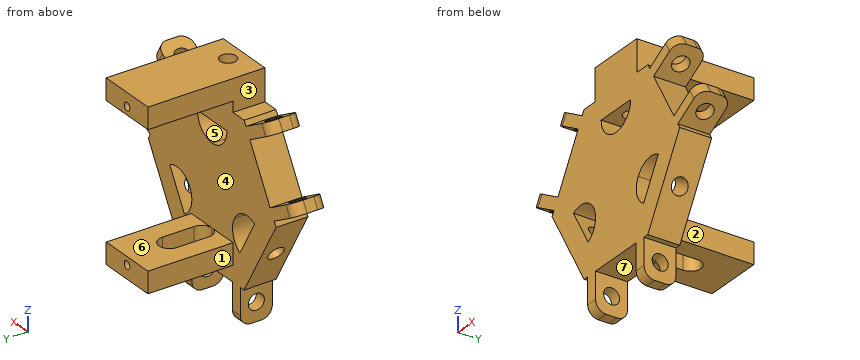
from build123d import *

# Parameters (mm, degrees)
BOSS_EXTRUDE1_DEPTH = 6
SKETCH2_W           = 2.16
SKETCH2_H           = 6
BOSS_EXTRUDE2_DEPTH = 7
SKETCH4_W           = 2.16
SKETCH4_H           = 6
BOSS_EXTRUDE3_DEPTH = 7
SKETCH5_W           = 2.16
SKETCH5_H           = 6
BOSS_EXTRUDE4_DEPTH = 7
SKETCH6_W           = 2.16
SKETCH6_H           = 6
BOSS_EXTRUDE5_DEPTH = 7
SKETCH7_W           = 2.16
SKETCH7_H           = 6
BOSS_EXTRUDE6_DEPTH = 7
SKETCH9_W           = 2.16
SKETCH9_H           = 6
BOSS_EXTRUDE7_DEPTH = 7
SKETCH11_W          = 11.320508076
SKETCH11_H          = 22
BOSS_EXTRUDE8_DEPTH = 6
SKETCH13_W          = 11.320508076
SKETCH13_H          = 2
CUT_EXTRUDE1_DEPTH  = 16
SKETCH14_W          = 11.320508076
SKETCH14_H          = 4
BOSS_EXTRUDE9_DEPTH = 16
SKETCH22_W          = 4
SKETCH22_H          = 10
CUT_EXTRUDE8_DEPTH  = 4
SKETCH23_R          = 1.5
CUT_EXTRUDE9_DEPTH  = 44.598981412
SKETCH24_R          = 1.5
CUT_EXTRUDE10_DEPTH = 45.916354208
SKETCH25_R          = 1.5
CUT_EXTRUDE11_DEPTH = 45.285561147
SKETCH26_W          = 8
SKETCH26_H          = 4
CUT_EXTRUDE12_DEPTH = 6
FILLET1_R           = 4
CUT_EXTRUDE13_DEPTH = 6
FILLET2_R           = 4
CUT_EXTRUDE14_DEPTH = 6
FILLET3_R           = 4
SKETCH34_R          = 1.5
CUT_EXTRUDE15_DEPTH = 4
SKETCH35_R          = 1.5
CUT_EXTRUDE16_DEPTH = 4
SKETCH36_R          = 1.5
CUT_EXTRUDE17_DEPTH = 10
FILLET4_R           = 2
FILLET5_R           = 2
SKETCH37_R          = 0.75
CUT_EXTRUDE19_DEPTH = 5
SKETCH39_R          = 0.75
CUT_EXTRUDE20_DEPTH = 5
FILLET6_R           = 2


with BuildPart() as part:
    # Sketch1 → Boss-Extrude1 (new body)
    with BuildSketch(Plane(origin=(0, 0, 0), x_dir=(1, 0, 0), z_dir=(0, 1, 0))):
        Polygon((17.320508076, 0), (8.660254038, 15), (-8.660254038, 15), (-17.320508076, 0), (-8.660254038, -15), (8.660254038, -15), align=None)
    extrude(amount=BOSS_EXTRUDE1_DEPTH)

    # Sketch2 → Boss-Extrude2 (add)
    with BuildSketch(Plane(origin=(12.990381057, 0, 7.5), x_dir=(0.4999999999999997, 0, -0.8660254037844388), z_dir=(0.8660254037844389, 0, 0.49999999999999983))):
        with Locations((-6.580254038, 3)):
            Rectangle(SKETCH2_W, SKETCH2_H)
    extrude(amount=BOSS_EXTRUDE2_DEPTH)

    # Sketch4 → Boss-Extrude3 (add)
    with BuildSketch(Plane(origin=(12.990381057, 0, 7.5), x_dir=(0.4999999999999997, 0, -0.8660254037844388), z_dir=(0.8660254037844389, 0, 0.49999999999999983))):
        with Locations((6.580254038, 3)):
            Rectangle(SKETCH4_W, SKETCH4_H)
    extrude(amount=BOSS_EXTRUDE3_DEPTH)

    # Sketch5 → Boss-Extrude4 (add)
    with BuildSketch(Plane(origin=(-12.990381057, 0, 7.5), x_dir=(0.4999999999999999, 0, 0.8660254037844387), z_dir=(-0.8660254037844388, 0, 0.49999999999999994))):
        with Locations((-6.580254038, 3)):
            Rectangle(SKETCH5_W, SKETCH5_H)
    extrude(amount=BOSS_EXTRUDE4_DEPTH)

    # Sketch6 → Boss-Extrude5 (add)
    with BuildSketch(Plane(origin=(-12.990381057, 0, 7.5), x_dir=(0.4999999999999999, 0, 0.8660254037844387), z_dir=(-0.8660254037844388, 0, 0.49999999999999994))):
        with Locations((6.580254038, 3)):
            Rectangle(SKETCH6_W, SKETCH6_H)
    extrude(amount=BOSS_EXTRUDE5_DEPTH)

    # Sketch7 → Boss-Extrude6 (add)
    with BuildSketch(Plane(origin=(0, 0, -15), x_dir=(-1, 0, 0), z_dir=(0, 0, -1))):
        with Locations((-6.580254038, 3)):
            Rectangle(SKETCH7_W, SKETCH7_H)
    extrude(amount=BOSS_EXTRUDE6_DEPTH)

    # Sketch9 → Boss-Extrude7 (add)
    with BuildSketch(Plane(origin=(0, 0, -15), x_dir=(-1, 0, 0), z_dir=(0, 0, -1))):
        with Locations((6.580254038, 3)):
            Rectangle(SKETCH9_W, SKETCH9_H)
    extrude(amount=BOSS_EXTRUDE7_DEPTH)

    # Sketch11 → Boss-Extrude8 (add)
    with BuildSketch(Plane.XY.offset(15)):
        with Locations((0, 11)):
            Rectangle(SKETCH11_W, SKETCH11_H)
    extrude(amount=BOSS_EXTRUDE8_DEPTH)

    # Sketch13 → Cut-Extrude1 (cut)
    with BuildSketch(Plane(origin=(0, 22, 0), x_dir=(1, 0, 0), z_dir=(0, 1, 0))):
        with Locations((0, -16)):
            Rectangle(SKETCH13_W, SKETCH13_H)
    extrude(amount=-CUT_EXTRUDE1_DEPTH, mode=Mode.SUBTRACT)

    # Sketch14 → Boss-Extrude9 (add)
    with BuildSketch(Plane(origin=(0, 6, 0), x_dir=(1, 0, 0), z_dir=(0, 1, 0))):
        with Locations((0, 10)):
            Rectangle(SKETCH14_W, SKETCH14_H)
    extrude(amount=BOSS_EXTRUDE9_DEPTH)

    # Sketch22 → Cut-Extrude8 (cut)
    with BuildSketch(Plane(origin=(0, 0, -12), x_dir=(-1, 0, 0), z_dir=(0, 0, -1))):
        with Locations((0.000254038, 11)):
            Rectangle(SKETCH22_W, SKETCH22_H)
    extrude(amount=-CUT_EXTRUDE8_DEPTH, mode=Mode.SUBTRACT)

    # Sketch23 → Cut-Extrude9 (cut, through all)
    with BuildSketch(Plane(origin=(7.660254038, 0, 0), x_dir=(0, 0, -1), z_dir=(1, 0, 0))):
        with Locations(Location((18.5, 3, 0), (0, 0, 90))):
            Circle(SKETCH23_R)
    extrude(amount=-CUT_EXTRUDE9_DEPTH, mode=Mode.SUBTRACT)

    # Sketch24 → Cut-Extrude10 (cut, through all)
    with BuildSketch(Plane(origin=(-3.830127019, 0, 6.633974596), x_dir=(0.8660254037844388, 0, 0.4999999999999997), z_dir=(-0.49999999999999983, 0, 0.8660254037844389))):
        with Locations((18.5, 3)):
            Circle(SKETCH24_R)
    extrude(amount=-CUT_EXTRUDE10_DEPTH, mode=Mode.SUBTRACT)

    # Sketch25 → Cut-Extrude11 (cut, through all)
    with BuildSketch(Plane(origin=(-3.830127019, 0, -6.633974596), x_dir=(-0.8660254037844387, 0, 0.4999999999999999), z_dir=(-0.4999999999999999, 0, -0.8660254037844387))):
        with Locations((18.5, 3)):
            Circle(SKETCH25_R)
    extrude(amount=-CUT_EXTRUDE11_DEPTH, mode=Mode.SUBTRACT)

    # Sketch26 → Cut-Extrude12 (cut)
    with BuildSketch(Plane(origin=(0, 6, 0), x_dir=(1, 0, 0), z_dir=(0, 1, 0))):
        with Locations((-0.000254038, -9)):
            Rectangle(SKETCH26_W, SKETCH26_H)
    extrude(amount=-CUT_EXTRUDE12_DEPTH, mode=Mode.SUBTRACT)

    # Fillet1
    fillet1_edges = [part.edges().sort_by_distance(p)[0] for p in [
        (-4.000254038, 3, 7),
        (3.999745962, 3, 7),
    ]]
    fillet(fillet1_edges, radius=FILLET1_R - 0.0001)  # a hair under: the kernel refuses the full size

    # Sketch32 → Cut-Extrude13 (cut)
    with BuildSketch(Plane(origin=(0, 6, 0), x_dir=(1, 0, 0), z_dir=(0, 1, 0))):
        Polygon((7.526152423, 8.964321618), (4.062050808, 6.964321618), (8.062304845, 0.035678382), (11.526406461, 2.035678382), align=None)
    extrude(amount=-CUT_EXTRUDE13_DEPTH, mode=Mode.SUBTRACT)

    # Fillet2
    fillet2_edges = [part.edges().sort_by_distance(p)[0] for p in [
        (8.062304845, 3, -0.035678382),
        (4.062050808, 3, -6.964321618),
    ]]
    fillet(fillet2_edges, radius=FILLET2_R - 0.0001)  # a hair under: the kernel refuses the full size

    # Sketch33 → Cut-Extrude14 (cut)
    with BuildSketch(Plane(origin=(0, 6, 0), x_dir=(1, 0, 0), z_dir=(0, 1, 0))):
        Polygon((-7.526406461, 8.963881612), (-11.526406461, 2.035678382), (-8.062304845, 0.035678382), (-4.062304845, 6.963881612), align=None)
    extrude(amount=-CUT_EXTRUDE14_DEPTH, mode=Mode.SUBTRACT)

    # Fillet3
    fillet3_edges = [part.edges().sort_by_distance(p)[0] for p in [
        (-8.062304845, 3, -0.035678382),
        (-4.062304845, 3, -6.963881612),
    ]]
    fillet(fillet3_edges, radius=FILLET3_R - 0.0001)  # a hair under: the kernel refuses the full size

    # Sketch34 → Cut-Extrude15 (cut)
    with BuildSketch(Plane(origin=(-12.990381057, 0, -7.5), x_dir=(-0.5, 0, 0.8660254037844386), z_dir=(-0.8660254037844387, 0, -0.5000000000000001))):
        with Locations((0, 3)):
            Circle(SKETCH34_R)
    extrude(amount=-CUT_EXTRUDE15_DEPTH, mode=Mode.SUBTRACT)

    # Sketch35 → Cut-Extrude16 (cut)
    with BuildSketch(Plane(origin=(12.990381057, 0, -7.5), x_dir=(-0.5000000000000003, 0, -0.8660254037844386), z_dir=(0.8660254037844385, 0, -0.5000000000000002))):
        with Locations((0, 3)):
            Circle(SKETCH35_R)
    extrude(amount=-CUT_EXTRUDE16_DEPTH, mode=Mode.SUBTRACT)

    # Sketch36 → Cut-Extrude17 (cut)
    with BuildSketch(Plane.XY.offset(21)):
        with Locations((0, 3)):
            Circle(SKETCH36_R)
    extrude(amount=-CUT_EXTRUDE17_DEPTH, mode=Mode.SUBTRACT)

    # Fillet4
    fillet4_edges = [part.edges().sort_by_distance(p)[0] for p in [
        (1.999745962, 16, -10),
        (-2.000254038, 16, -10),
    ]]
    fillet(fillet4_edges, radius=FILLET4_R - 0.0001)  # a hair under: the kernel refuses the full size

    # Fillet5
    fillet5_edges = [part.edges().sort_by_distance(p)[0] for p in [
        (1.999745962, 6, -10),
        (-2.000254038, 6, -10),
    ]]
    fillet(fillet5_edges, radius=FILLET5_R - 0.0001)  # a hair under: the kernel refuses the full size

    # Sketch37 → Cut-Extrude19 (cut)
    with BuildSketch(Plane(origin=(0, 22, 0), x_dir=(1, 0, 0), z_dir=(0, 1, 0))):
        with Locations(Location((0, 9.5, 0), (0, 0, 270))):
            Circle(SKETCH37_R)
    extrude(amount=-CUT_EXTRUDE19_DEPTH, mode=Mode.SUBTRACT)

    # Sketch39 → Cut-Extrude20 (cut)
    with BuildSketch(Plane(origin=(0, 22, 0), x_dir=(1, 0, 0), z_dir=(0, 1, 0))):
        with Locations(Location((0, -18.5, 0), (0, 0, 270))):
            Circle(SKETCH39_R)
    extrude(amount=-CUT_EXTRUDE20_DEPTH, mode=Mode.SUBTRACT)

    # Fillet6
    fillet6_edges = [part.edges().sort_by_distance(p)[0] for p in [
        (15.762431864, 6, 16.69866716),
        (15.762431864, 0, 16.69866716),
        (22.342685902, 0, 5.30133284),
        (22.342685902, 6, 5.30133284),
        (-22.342685902, 0, 5.30133284),
        (-22.342685902, 6, 5.30133284),
        (-15.762431864, 0, 16.69866716),
        (-15.762431864, 6, 16.69866716),
        (6.580254038, 6, -22),
        (6.580254038, 0, -22),
        (-6.580254038, 0, -22),
        (-6.580254038, 6, -22),
    ]]
    fillet(fillet6_edges, radius=FILLET6_R)


solid = part.part
Read the model definition and answer for the solid it produces. Units are mm, in the model's axes. Face numbers are marked on the shaded views. A direction names the side the tool comes from. Give positions to 0.01 mm unless a question says otherwise; leave off trailing zeros. Write each loop counter-clockwise with the first axis right and the second up, starting at its lowest first coordinate (ties: lowest second). Pieces come first, ordered by that corner, then holes. Notation, with made-up numbers: M 6.25,-22.75 L 43.25,-22.75 A13 cw 43.25,-17.75 Z; hole C 9,59 d1. An arc over 180 degrees is marked long. One line per item, written item: value. Start each with the question number.
(1) Find section C-C (z = 18.5). Determine the outline of the cut face in (x, y).
(2) Find section D-D (y = 9.75). Determine the outline of the cut face in (x, z).
(3) Determine the mould class of the marked faces 1, 2, 3 and 4 for opening direction X: pulls with the +X half, pulls with the -X half, needs draft (parallel to the pull), parting line crosses it, or undercut.
(4) Find section A-A (z = -16). Determine the outline of the cut face in (x, y), plus the area to 3 significant figures.
(5) Find section B-B (y = 18.75). Determine the outline of the cut face in (x, z), plus the area to 3 significant figures.
(6) Find the intervals of material crossed by line 1 (Y direction, x = 0, z = 16); line 2 (Z direction, x = 6.45, y = 3); line 3 (Z direction, x = -1, y = 19.75), in increasing order.
(7) A tool of negligible diameter and unlimited length cuts with its end or side. For the marked faces 5, 6 and 7, from which of +Z, -Z, +X, -X, +Y, -Y can it reach the whole face along a straight path? Write none if from no direction.
(8) Flat-ended cylindrical pins translate along their axes: pin 1 Ø3 at (x, y) = (-1, 4.5) entering from -Z; pin 2 Ø2.5 at (x, y) = (0, 3) entering from +Z; pin 3 Ø3 at (y, z) = (11, -9.5) entering from +X; pin 4 Ø10 at (y, z) = (14.5, 11) entering from -X. Find the tip coordinate at first contact, or state that the pin passes through.
Results below:
1. outline: M -5.66,0 L 5.66,0 L 5.66,22 L 0.75,22 L 0.75,17 L -0.75,17 L -0.75,22 L -5.66,22 Z; hole C 0,3 d3
2. outline: M -5.66,-12 L -2,-12 L -2,-8 L -5.66,-8 Z; M -5.66,17 L 5.66,17 L 5.66,21 L -5.66,21 Z; M 2,-12 L 5.66,-12 L 5.66,-8 L 2,-8 Z
3. face 1: pulls with the -X half
3. face 2: pulls with the +X half
3. face 3: undercut
3. face 4: needs draft
4. outline: M -7.66,0 L -5.5,0 L -5.5,6 L -7.66,6 Z; M 5.5,0 L 7.66,0 L 7.66,6 L 5.5,6 Z
4. area: 25.9 mm^2
5. outline: M -5.66,-12 L 5.66,-12 L 5.66,-8 L -5.66,-8 Z; M -5.66,17 L 5.66,17 L 5.66,21 L -5.66,21 Z; hole C 0,-9.5 d1.5; hole C 0,18.5 d1.5
5. area: 87.0 mm^2
6. line 1: y = 0 to 1.5, 4.5 to 6
6. line 2: z = -22 to -20, -17 to -8.06, -2.94 to 15
6. line 3: z = -12 to -8, 17 to 21
7. face 5: +Y, -Y
7. face 6: +X, -X, +Y
7. face 7: -Z, +Y, -Y
8. pin 1: stops at z = -15
8. pin 2: stops at z = 7.2
8. pin 3: stops at x = 5.66
8. pin 4: passes through
